Here's how the part is built. I have some questions about the finished solid (model axes, mm). A direction names the side the tool comes from. Give positions to 0.01 mm unless a question says otherwise; leave off trailing zeros. Write each loop counter-clockwise with the first axis right and the second up, starting at its lowest first coordinate (ties: lowest second). Pieces come first, ordered by that corner, then holes. Notation, with made-up numbers: (54.5, -6) - (60.5, -6) arc R23 ccw to (60.5, 7) - close; hole circle Ø5 at (25.5, -14.75). An arc over 180 degrees is marked (long way). One line per item, written item: value. Start each with the question number.
1) Imagine slicing it at A-A on z = 6. Write out the boundary of the cut face in (x, y), plus the area to 3 significant figures.
2) Imagine slicing it at B-B on y = 13. Write out the boundary of the cut face in (x, z).
3) Please list where these lines run through material, in increasing order: L1, parallel to X at y = 0, z = 5.5; L2, parallel to Y at x = 15, z = 0.75. Write a range as [from, to].
4) On a 3-axis mill with a long thin cutter (end or side, diameter ignored), from which of +Z, -Z, +X, -X, +Y, -Y can I reach the whole of each face in a straight line? I mean faces 1 (the flat face through (14, -12.573, 1)), 2 (the flat face through (-14, -8.509, 1)), 3 (the flat face through (-15, 28, 1.524)), 4 (the flat face through (14, 26.035, 1)). Say none if no direction works.
5) We'd pull the mould along Y, two halves only. Please class faces 5 (the flat face through (-14, -12.573, 1)), 6 (the cylindrical face through (-16.764, -10.586, 0.751)), 7 (the cylindrical face through (16.764, -10.496, 0.751)), 8 (the flat face through (15, -11, 1.524)): +Y half, -Y half, draft (parallel to the pull), parting line (faces both ways), or undercut.
6) I'm going to push flat-ended pins straight in: P1, Ø2, axis at x = -14.5, y = 28, coming from the +Z side; P2, Ø6, axis at y = -7.5, z = 8.5, coming from the -X side; P3, Ø0.8, axis at x = 13.5, z = 1, coming from the -Y side. Where does each tip first touch, or does it pass through?
Autodesk Inventor part; units mm, degrees
ref_plane "YZ Plane" through (0, 0, 0) normal (1, 0, 0) x (0, 1, 0)
ref_plane "XZ Plane" through (0, 0, 0) normal (0, 1, 0) x (-1, 0, 0)
ref_plane "XY Plane" through (0, 0, 0) normal (0, 0, 1) x (1, 0, 0)
sketch "Sketch1" plane through (0, 0, 0) normal (0, 0, 1) x (1, 0, 0)
  line L0 (12.7, 30.099) -> (-12.7, 30.099)
  line L1 (-12.7, 30.099) -> (-12.7, -30.099)
  line L2 (-12.7, -30.099) -> (12.7, -30.099)
  line L3 (12.7, -30.099) -> (12.7, 30.099)
  point P0 (0, 0)
  point P1 (0, 30.099)
  point P2 (-12.7, 0)
  dimension "d0" = 60.198
  dimension "d1" = 25.4
extrude "Extrusion1" add sketch "Sketch1" along normal blind 10.16
sketch "Sketch2" plane through (0, 0, 0) normal (0, 0, -1) x (-1, 0, 0)
  line L0 (-12.7, 30.099) -> (12.7, 30.099)
  line L1 (-12.7, -30.099) -> (-12.7, 30.099)
  line L2 (12.7, -30.099) -> (-12.7, -30.099)
  arc A0 (-14.732, 30.099) -> (-14.732, 26.035) centre (-14.732, 28.067) ccw
  line L3 (-14.732, 30.099) -> (-12.7, 30.099)
  line L4 (-14.732, 26.035) -> (-12.7, 26.035)
  line L5 (0, 30.099) -> (0, -30.099)
  arc A1 (-14.732, -8.509) -> (-14.732, -12.573) centre (-14.732, -10.541) ccw
  line L6 (-14.732, -8.509) -> (-12.7, -8.509)
  line L7 (-14.732, -12.573) -> (-12.7, -12.573)
  line L8 (-12.7, 30.099) -> (-12.7, 26.035)
  line L9 (-12.7, -8.509) -> (-12.7, -12.573)
  arc A2 (14.732, 26.035) -> (14.732, 30.099) centre (14.732, 28.067) ccw
  line L10 (14.732, 30.099) -> (12.7, 30.099)
  line L11 (14.732, 26.035) -> (12.7, 26.035)
  arc A3 (14.732, -12.573) -> (14.732, -8.509) centre (14.732, -10.541) ccw
  line L12 (14.732, -8.509) -> (12.7, -8.509)
  line L13 (14.732, -12.573) -> (12.7, -12.573)
  line L14 (12.7, 30.099) -> (12.7, 26.035)
  line L15 (12.7, -8.509) -> (12.7, -12.573)
  point P0 (0, 0)
  dimension "d4" = 2.032
  dimension "d5" = 2.032
  dimension "d6" = 42.672
extrude "Extrusion2" add sketch "Sketch2" against normal blind 1.524 contours L10 A2 L11 L14 | L1 L4 A0 L3 | L1 L7 A1 L6 | L13 L15 L12 A3
properties part number "Lisa-M"
Numbers:
1. outline: (-12.7, -30.1) - (12.7, -30.1) - (12.7, 30.1) - (-12.7, 30.1) - close
1. area: 1,530 mm^2
2. outline: (-12.7, 0) - (12.7, 0) - (12.7, 10.16) - (-12.7, 10.16) - close
3. L1: [-12.7, 12.7]
3. L2: [-12.56, -8.53], [26.05, 30.08]
4. face 1: +Z, -Z, +X, -Y
4. face 2: +Z, -Z, -X
4. face 3: +Z, -X, +Y, -Y
4. face 4: +Z, -Z, +X
5. face 5: -Y half
5. face 6: undercut
5. face 7: undercut
5. face 8: draft
6. P1: z = 1.52
6. P2: x = -12.7
6. P3: y = -12.57
